Work out the finished part from the listing and answer in its coordinate system (mm). A direction names the side the tool comes from. Give positions to 0.01 mm unless a question says otherwise; leave off trailing zeros. Loops run counter-clockwise (first coordinate to the right, second up) from the corner with the lowest first, then second, coordinate; pieces in that order, holes last. Notation, with made-up numbers: (29, -4) - (51, -4) arc R14 cw to (51, 15) - close; hole circle Ø9 at (53.5, -15). An arc over 180 degrees is marked (long way). Use CSV: the item, a comma, the result in double quotes.
from build123d import *

# Parameters (mm, degrees)
SKETCH10_R           = 25
SKETCH10_R_2         = 12.5
BOSS_EXTRUDE7_DEPTH  = 33
BOSS_EXTRUDE9_START  = 5
BOSS_EXTRUDE9_DEPTH  = 56
SKETCH13_R           = 8
CUT_EXTRUDE1_DEPTH   = 16
BOSS_EXTRUDE12_DEPTH = 17
SKETCH17_R           = 6
CUT_EXTRUDE2_DEPTH   = 17
BOSS_EXTRUDE13_DEPTH = 12
SKETCH20_R           = 8
CUT_EXTRUDE3_DEPTH   = 27
FILLET1_R            = 2


with BuildPart() as part:
    # Sketch10 → Boss-Extrude7 (new, symmetric)
    with BuildSketch(Plane.XY):
        Circle(SKETCH10_R)
        Circle(SKETCH10_R_2, mode=Mode.SUBTRACT)
    extrude(amount=BOSS_EXTRUDE7_DEPTH, both=True)



with BuildPart() as body_2:
    # Sketch12 → Boss-Extrude9 (new body)
    with BuildSketch(Plane(origin=(0, 0, 33), x_dir=(-1, 0, 0), z_dir=(0, 0, -1)).offset(BOSS_EXTRUDE9_START)):
        with BuildLine():
            Line((0, -36), (75, -36))
            Line((75, -36), (75, -20))
            Line((75, -20), (27, -20))
            ThreePointArc((27, -20), (25.585786438, -19.414213562), (25, -18))
            Line((25, -18), (25, 0))
            ThreePointArc((25, 0), (0, -25), (-25, 0))
            Line((-25, 0), (-25, -7))
            ThreePointArc((-25, -7), (-25.585786438, -8.414213562), (-27, -9))
            Line((-27, -9), (-90, -9))
            Line((-90, -9), (-90, -36))
            Line((-90, -36), (0, -36))
        make_face()
    extrude(amount=BOSS_EXTRUDE9_DEPTH)

    # Sketch13 → Cut-Extrude1 (cut)
    with BuildSketch(Plane(origin=(0, -20, 0), x_dir=(1, 0, 0), z_dir=(0, 1, 0))):
        with Locations(Location((-50, 3, 0), (0, 0, 270))):
            Circle(SKETCH13_R)
    extrude(amount=-CUT_EXTRUDE1_DEPTH, mode=Mode.SUBTRACT)


with BuildPart() as body_3:
    # Sketch15 → Boss-Extrude12 (new body)
    with BuildSketch(Plane.XY.offset(33)):
        with BuildLine():
            ThreePointArc((60, 0), (42.426406871, 42.426406871), (0, 60))
            ThreePointArc((0, 60), (-15, 75), (0, 90))
            ThreePointArc((0, 90), (63.639610307, 63.639610307), (90, 0))
            ThreePointArc((90, 0), (75, -15), (60, 0))
        make_face()
    extrude(amount=-BOSS_EXTRUDE12_DEPTH)

    # Sketch17 → Cut-Extrude2 (cut)
    with BuildSketch(Plane.XY.offset(33)):
        with Locations((0, 75)):
            Circle(SKETCH17_R)
        with Locations((37.5, 64.951905284)):
            Circle(SKETCH17_R)
        with Locations((64.951905284, 37.5)):
            Circle(SKETCH17_R)
        with Locations((75, 0)):
            Circle(SKETCH17_R)
    extrude(amount=-CUT_EXTRUDE2_DEPTH, mode=Mode.SUBTRACT)


with BuildPart() as part_1:
    add(part.part)

    add(body_2.part)  # Boss-Extrude13 merges body 2

    add(body_3.part)  # Boss-Extrude13 merges body 3
    # Sketch18 → Boss-Extrude13 (add)
    with BuildSketch(Plane.XY.offset(28)):
        with BuildLine():
            Line((25, -7), (58, -7))
            ThreePointArc((58, -7), (59.414213562, -6.414213562), (60, -5))
            Line((60, -5), (60, 0))
            ThreePointArc((60, 0), (60.769750529, -4.74341649), (63, -9))
            Line((63, -9), (27, -9))
            ThreePointArc((27, -9), (25.585786438, -8.414213562), (25, -7))
        make_face()
        with BuildLine():
            Line((-15, 75), (-15, 20))
            ThreePointArc((-15, 20), (0, 25), (15, 20))
            Line((15, 20), (15, 58.094750193))
            ThreePointArc((15, 58.094750193), (7.560257549, 59.521781776), (0, 60))
            ThreePointArc((0, 60), (-10.606601718, 64.393398282), (-15, 75))
        make_face()
    extrude(amount=-BOSS_EXTRUDE13_DEPTH)

    # Sketch20 → Cut-Extrude3 (cut)
    with BuildSketch(Plane(origin=(0, -9, 0), x_dir=(1, 0, 0), z_dir=(0, 1, 0))):
        with Locations(Location((57.5, 3, 0), (0, 0, 270))):
            Circle(SKETCH20_R)
    extrude(amount=-CUT_EXTRUDE3_DEPTH, mode=Mode.SUBTRACT)

    # Fillet1
    fillet1_edges = [part_1.edges().sort_by_distance(p)[0] for p in [
        (-15, 20, 22),
    ]]
    fillet(fillet1_edges, radius=FILLET1_R)


solid = part_1.part
Item 1: Given P1, Ø1.5, axis at y = -2, z = 19.5, coming from the -X side; P2, Ø3, axis at x = 70, z = 11, coming from the +Y side; P3, Ø3.5, axis at y = -3.5, z = 12, coming from the +X side, each flat-ended and moving along its own axis, determine where each tip first touches the part or whether it passes through.
Determined:
P1,"stops at x = -25"
P2,"stops at y = -9"
P3,"stops at x = 25"
Item 2: For faces 1 (the flat face through (-15, 48, 22)), 2 (the flat face through (-75, -28, 0)), 3 (the flat face through (15, 39, 22)), determine the directions among +Z, -Z, +X, -X, +Y, -Y from which every point of the face is accessible in a straight line to the end or side of a thin tool.
Determined:
face 1,"+Z, -Z, -X, +Y"
face 2,"+Z, -Z, -X, +Y, -Y"
face 3,"+Z, -Z"
Item 3: The mould has two halves that part along Z. Classify faces 4 (the flat face through (-1, 41, 28)), 5 (the cylindrical face through (65.432, -22.311, -4.041)), 6 (the flat face through (9, -36, 0)): pulls with the +Z half, pulls with the -Z half, needs draft (parallel to the pull), parting line crosses it, or undercut.
Determined:
face 4,"pulls with the +Z half"
face 5,"undercut"
face 6,"needs draft"
Item 4: Find the intervals of material crossed by line 1 (X direction, y = -26, z = -3); line 2 (X direction, y = 7.5, z = 30); line 3 (X direction, y = 15, z = 10.5), in increasing order.
Determined:
line 1,"x = -75 to -58, -42 to 49.5, 65.5 to 90"
line 2,"x = -23.85 to -10, 10 to 23.85, 59.53 to 89.69"
line 3,"x = -20 to 20"
Item 5: A cutting plane is placed at A-A on z = -3. Determine the outline of the cut face in (x, y).
Determined:
outline,"(-75, -36) - (-58, -36) - (-58, -20) - (-75, -20) - close; (-42, -36) - (49.5, -36) - (49.5, -9) - (27, -9) arc R2 cw to (25, -7) - (25, 0) arc R25 ccw to (-25, 0) - (-25, -18) arc R2 cw to (-27, -20) - (-42, -20) - close; (65.5, -36) - (90, -36) - (90, -9) - (65.5, -9) - close; hole circle Ø25 at (0, 0)"
Item 6: A cutting plane is placed at C-C on x = 37.5. Determine the outline of the cut face in (y, z).
Determined:
outline,"(-36, -28) - (-9, -28) - (-9, 16) - (-7, 16) - (-7, 28) - (-36, 28) - close; (46.84, 16) - (58.95, 16) - (58.95, 33) - (46.84, 33) - close; (70.95, 16) - (81.82, 16) - (81.82, 33) - (70.95, 33) - close"
Item 7: A cutting plane is placed at D-D on z = -20. Determine the outline of the cut face in (x, y).
Determined:
outline,"(-75, -36) - (90, -36) - (90, -9) - (27, -9) arc R2 cw to (25, -7) - (25, 0) arc R25 ccw to (-25, 0) - (-25, -18) arc R2 cw to (-27, -20) - (-75, -20) - close; hole circle Ø25 at (0, 0)"
Item 8: A cutting plane is placed at B-B on y = -2.5. Determine the outline of the cut face in (x, z), and give its area (3 significant figures).
Determined:
outline,"(-25, -28) - (-24.87, -28) - (-24.87, -33) - (-12.25, -33) - (-12.25, 33) - (-24.87, 33) - (-24.87, 28) - (-25, 28) - close; (12.25, -33) - (24.87, -33) - (24.87, -28) - (25, -28) - (25, 28) - (24.87, 28) - (24.87, 33) - (12.25, 33) - close; (60, 16) - (69.55, 16) - (69.55, 33) - (60.21, 33) - (60.21, 28) - (60, 28) - close; (80.45, 16) - (89.79, 16) - (89.79, 33) - (80.45, 33) - close"
area,"2,000 mm²"
